from build123d import *

# Parameters (mm, degrees)
SKETCH1_W               = 45
SKETCH1_H               = 70
BOSS_EXTRUDE1_DEPTH     = 10
SKETCH2_W               = 20.25
SKETCH2_H               = 5.1
CUT_EXTRUDE1_DEPTH      = 1
CUT_EXTRUDE1_DEPTH_BACK = 46
SKETCH3_R               = 4.15
CUT_EXTRUDE2_DEPTH      = 11
SKETCH5_R               = 4.15
BOSS_EXTRUDE2_DEPTH     = 10
CHAMFER1_SIZE           = 1
CHAMFER1_SIZE2          = 1.191753593


with BuildPart() as part:
    # Sketch1 → Boss-Extrude1 (new body)
    with BuildSketch(Plane(origin=(0, 0, 0), x_dir=(1, 0, 0), z_dir=(0, 1, 0))):
        Rectangle(SKETCH1_W, SKETCH1_H)
    extrude(amount=BOSS_EXTRUDE1_DEPTH)

    # Sketch2 → Cut-Extrude1 (cut, two sides)
    with BuildSketch(Plane(origin=(22.5, 0, 0), x_dir=(0, 0, -1), z_dir=(1, 0, 0))) as cut_extrude1_sk:
        with Locations((0, 2.55)):
            Rectangle(SKETCH2_W, SKETCH2_H)
    extrude(amount=CUT_EXTRUDE1_DEPTH, mode=Mode.SUBTRACT)
    extrude(cut_extrude1_sk.sketch, amount=-CUT_EXTRUDE1_DEPTH_BACK, mode=Mode.SUBTRACT)

    # Sketch3 → Cut-Extrude2 (cut, through all)
    with BuildSketch(Plane.XZ):
        with Locations((15, 25)):
            Circle(SKETCH3_R)
        with Locations((15, -25)):
            Circle(SKETCH3_R)
        with Locations((-15, -25)):
            Circle(SKETCH3_R)
        with Locations((-15, 25)):
            Circle(SKETCH3_R)
    extrude(amount=-CUT_EXTRUDE2_DEPTH, mode=Mode.SUBTRACT)

    # Sketch5 → Boss-Extrude2 (add)
    with BuildSketch(Plane(origin=(0, 10, 0), x_dir=(1, 0, 0), z_dir=(0, 1, 0))):
        Polygon((-5.15, -35), (-22.5, -35), (-22.5, 35), (22.5, 35), (22.5, -35), (5.15, -35), (5.130229348, -34.949305848), (5.15, 31), (-5.15, 31), align=None)
        with Locations((-15, 25)):
            Circle(SKETCH5_R, mode=Mode.SUBTRACT)
        with Locations((15, 25)):
            Circle(SKETCH5_R, mode=Mode.SUBTRACT)
        with Locations((15, -25)):
            Circle(SKETCH5_R, mode=Mode.SUBTRACT)
        with Locations((-15, -25)):
            Circle(SKETCH5_R, mode=Mode.SUBTRACT)
    extrude(amount=BOSS_EXTRUDE2_DEPTH)

    # Chamfer1
    chamfer1_edges = [part.edges().sort_by_distance(p)[0] for p in [
        (-19.15, 20, -25),
        (10.85, 20, -25),
        (10.85, 20, 25),
        (-19.15, 20, 25),
    ]]
    chamfer1_side = [part.faces().sort_by_distance(p)[0] for p in [
        (-13.825, 20, 34.167834151),
    ]]
    chamfer(chamfer1_edges, length=CHAMFER1_SIZE, length2=CHAMFER1_SIZE2, reference=chamfer1_side[0])


solid = part.part
CAD build for the part. Positions are in the model's coordinates, mm. A direction names the side the tool comes from. Coordinates: 2 decimals unless noted, no trailing zeros. Loops run counter-clockwise (first coordinate to the right, second up) from the corner with the lowest first, then second, coordinate; pieces in that order, holes last. Notation, with made-up numbers: (79, 23.5) -> (84, 23.5) arc R17 cw to (84, 36.5) -> close; hole circle Ø3 at (6.25, 21.25). An arc over 180 degrees is marked (long way). One line per item, written item: value.
1. Slice it at A-A on x = 15. Write the cut outline in (y, z) (3 decimals).
Answers:
outline: (0, -35) -> (20, -35) -> (20, -30.15) -> (18.808, -29.15) -> (0, -29.15) -> close; (0, -20.85) -> (18.808, -20.85) -> (20, -19.85) -> (20, 19.85) -> (18.808, 20.85) -> (0, 20.85) -> (0, 10.125) -> (5.1, 10.125) -> (5.1, -10.125) -> (0, -10.125) -> close; (0, 29.15) -> (18.808, 29.15) -> (20, 30.15) -> (20, 35) -> (0, 35) -> close
2. Which spindle directions (+Z, -Z, +X, -X, +Y, -Y) get a long thin tool onto all of the face, cutting with end or side? Do faces 1 (the face through (0, 3, -10.125)), 2 (the face through (14.1, 9.27, -20.95)), 3 (the face through (0, 15, -31)). Say none if no direction does.
Answers:
face 1: +X, -X, -Y
face 2: +Y, -Y
face 3: +Z, +Y
3. Slice it at C-C on z = -25. Write the cut outline in (x, y), and give its area (3 significant figures).
Answers:
outline: (-22.5, 0) -> (-19.15, 0) -> (-19.15, 18.81) -> (-20.15, 20) -> (-22.5, 20) -> close; (-10.85, 0) -> (10.85, 0) -> (10.85, 18.81) -> (9.85, 20) -> (5.15, 20) -> (5.15, 10) -> (-5.15, 10) -> (-5.15, 20) -> (-9.85, 20) -> (-10.85, 18.81) -> close; (19.15, 0) -> (22.5, 0) -> (22.5, 20) -> (20.15, 20) -> (19.15, 18.81) -> close
area: 463 mm^2
4. Flat gauge pins, fed straight in: P1, Ø3, axis at x = -16, z = 23, coming from the -Y side; P2, Ø10, axis at x = 0.5, z = -2, coming from the -Y side; P3, Ø9.5, axis at x = 15, z = -25, coming from the +Y side; P4, Ø3, axis at x = 1, y = 14, coming from the +Z side. Where does each tip first touch, or does it go through?
Answers:
P1: passes through
P2: stops at y = 5.1
P3: stops at y = 19.52
P4: stops at z = -31
5. Slice it at D-D on x = 1.5. Write the cut outline in (y, z) (3 decimals).
Answers:
outline: (0, -35) -> (20, -35) -> (20, -31) -> (10, -31) -> (10, 35) -> (0, 35) -> (0, 10.125) -> (5.1, 10.125) -> (5.1, -10.125) -> (0, -10.125) -> close
6. Drill centre lines: line 1 (X direction, y = 6.5, z = -25); line 2 (Z direction, x = 6, y = 1.5) (3 decimals); line 3 (Z direction, x = 15, y = 5) (3 decimals). Where is each one in solid material? Low to high. Write a range as [from, to].
Answers:
line 1: x = [-22.5, -19.15], [-10.85, 10.85], [19.15, 22.5]
line 2: z = [-35, -10.125], [10.125, 35]
line 3: z = [-35, -29.15], [-20.85, -10.125], [10.125, 20.85], [29.15, 35]
7. Slice it at B-B on y = 2.25. Write the cut outline in (x, z) (3 decimals), and give its area (3 significant figures).
Answers:
outline: (-22.5, -35) -> (22.5, -35) -> (22.5, -10.125) -> (-22.5, -10.125) -> close; (-22.5, 10.125) -> (22.5, 10.125) -> (22.5, 35) -> (-22.5, 35) -> close; hole circle Ø8.3 at (-15, -25); hole circle Ø8.3 at (-15, 25); hole circle Ø8.3 at (15, -25); hole circle Ø8.3 at (15, 25)
area: 2,020 mm^2
8. Pull direction Z, two halves, no side cores. Call faces 4 (the face through (-22.5, 10, 0)), 5 (the face through (0, 8, 35)), 6 (the face through (0, 5.1, 0)): pulls with the +Z half, pulls with the -Z half, needs draft (parallel to the pull), parting line crosses it, or undercut.
Answers:
face 4: needs draft
face 5: pulls with the +Z half
face 6: undercut
